```python
from build123d import *

# Parameters (mm, degrees)
F0_W     = 175.5796000361
F0_H     = 94.5478640497
F1_DEPTH = 107.95
F2_W     = 77.0752280027
F2_H     = 175.5796000361
F3_DEPTH = 49.53
F4_W     = 54.9968387008
F4_H     = 113.6317700148
F5_DEPTH = 25.4


with BuildPart() as f1:
    # F0 (on Right) → F1 (new body)
    with BuildSketch(Plane.YZ):
        with Locations((5.5083744228, 4.4014062732)):
            Rectangle(F0_W, F0_H)
    extrude(amount=F1_DEPTH)

    # F2 (on face) → F3 (cut)
    with BuildSketch(Plane.XY.offset(51.6753382981)):
        with Locations((69.4123859987, 5.5083744228)):
            Rectangle(F2_W, F2_H)
    extrude(amount=-F3_DEPTH, mode=Mode.SUBTRACT)

    # F4 (on face) → F5 (cut)
    with BuildSketch(Plane.XY.offset(2.1453382981)):
        with Locations((80.4515806496, 8.1303864717)):
            Rectangle(F4_W, F4_H)
    extrude(amount=-F5_DEPTH, mode=Mode.SUBTRACT)


solid = f1.part
```
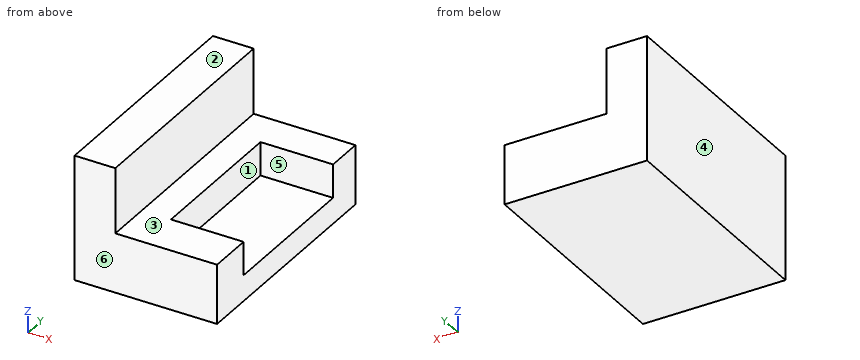
The model under review builds one solid part; all positions refer to its coordinate system, in mm. Face numbers are marked on the shaded views. A direction names the side the tool comes from. Coordinates: 2 decimals unless noted, no trailing zeros. Order: outer loops, then holes, each group sorted by start corner. A loop starts at its lowest first (then second) coordinate and runs counter-clockwise, first axis right, second up. Notation, with made-up numbers: (-17.5, -1.75) -> (5.5, -1.75) arc R20 ccw to (5.5, 25.25) -> close; hole circle Ø2 at (-33, -21). An arc over 180 degrees is marked (long way). Answer in a Markdown table with one row per item. Add a question column.
Item 1: Mouldability with a two-part tool opening along Y and no side actions: class the marked faces 4, 5 and 6 as +Y half, -Y half, draft (parallel to the pull), parting line (faces both ways), or undercut.
Item 2: Clearance check with flat-ended pins moving along their axes: pin 1 (20.5 mm diameter, centred on y = -11, z = -8, fed in from +X); pin 2 (12 mm diameter, centred on y = 15, z = 6.5, fed in from -X); pin 3 (2 mm diameter, centred on y = -10, z = 17.5, fed in from +X); pin 4 (4 mm diameter, centred on x = 34.5, z = 24.5, fed in from +Y). State where each tip first meets the part, or that it passes through.
Item 3: We need section B-B on x = 91.5. Write out the cut boundary in (y, z), plus the area to 3 significant figures.
Item 4: Machinability: for the marked faces 1, 2 and 3, which of the approach directions +Z, -Z, +X, -X, +Y, -Y give a long, thin tool a straight path to every point of the face, cutting with its end or side? Answer none if there is none.
Item 5: To check wall thickness, follow probe 1 along Y at (x, z) = (83, -18); probe 2 along Z at (x, y) = (100.5, -26); probe 3 along X at (y, z) = (-65.5, 21). State the ranges of each line that lie inside material, in increasing order.
Item 6: We need section C-C on z = -5. Write out the cut boundary in (x, y), plus the area to 3 significant figures.
Item 7: We need section D-D on x = 50.5. Write out the cut boundary in (y, z), plus the area to 3 significant figures.
Item 8: We need section A-A on y = 73. Write out the cut boundary in (x, z).
Final values:
| question | item | result |
|---|---|---|
| 1 | face 4 | draft |
| 1 | face 5 | undercut |
| 1 | face 6 | -Y half |
| 2 | pin 1 | stops at x = 52.95 |
| 2 | pin 2 | stops at x = 0 |
| 2 | pin 3 | stops at x = 30.87 |
| 2 | pin 4 | passes through |
| 3 | outline | (-82.28, -42.87) -> (93.3, -42.87) -> (93.3, 2.15) -> (64.95, 2.15) -> (64.95, -23.25) -> (-48.69, -23.25) -> (-48.69, 2.15) -> (-82.28, 2.15) -> close |
| 3 | area | 5,020 mm2 |
| 4 | face 1 | +Z, +X |
| 4 | face 2 | +Z, +X, -X, +Y, -Y |
| 4 | face 3 | +Z, +X, +Y, -Y |
| 5 | probe 1 | y = -82.28 to -48.69, 64.95 to 93.3 |
| 5 | probe 2 | z = -42.87 to -23.25 |
| 5 | probe 3 | x = 0 to 30.87 |
| 6 | outline | (0, -82.28) -> (107.95, -82.28) -> (107.95, -48.69) -> (52.95, -48.69) -> (52.95, 64.95) -> (107.95, 64.95) -> (107.95, 93.3) -> (0, 93.3) -> close |
| 6 | area | 12,700 mm2 |
| 7 | outline | (-82.28, -42.87) -> (93.3, -42.87) -> (93.3, 2.15) -> (-82.28, 2.15) -> close |
| 7 | area | 7,900 mm2 |
| 8 | outline | (0, -42.87) -> (107.95, -42.87) -> (107.95, 2.15) -> (30.87, 2.15) -> (30.87, 51.68) -> (0, 51.68) -> close |
